Check sheet for the drawn part. Datum: minimum x, y, z corner. Units: mm. A direction names the side the tool comes from. Give positions to 0.01 mm unless a question says otherwise; leave off trailing zeros. Order: outer loops, then holes, each group sorted by start corner. A loop starts at its lowest first (then second) coordinate and runs counter-clockwise, first axis right, second up. Notation, with made-up numbers: M 63.5,14 L 92.5,14 A23 ccw 92.5,45 Z; hole C 56.25,35 d6. An arc over 180 degrees is marked long. One line per question, with ' | ' between items. Start each with the question number.
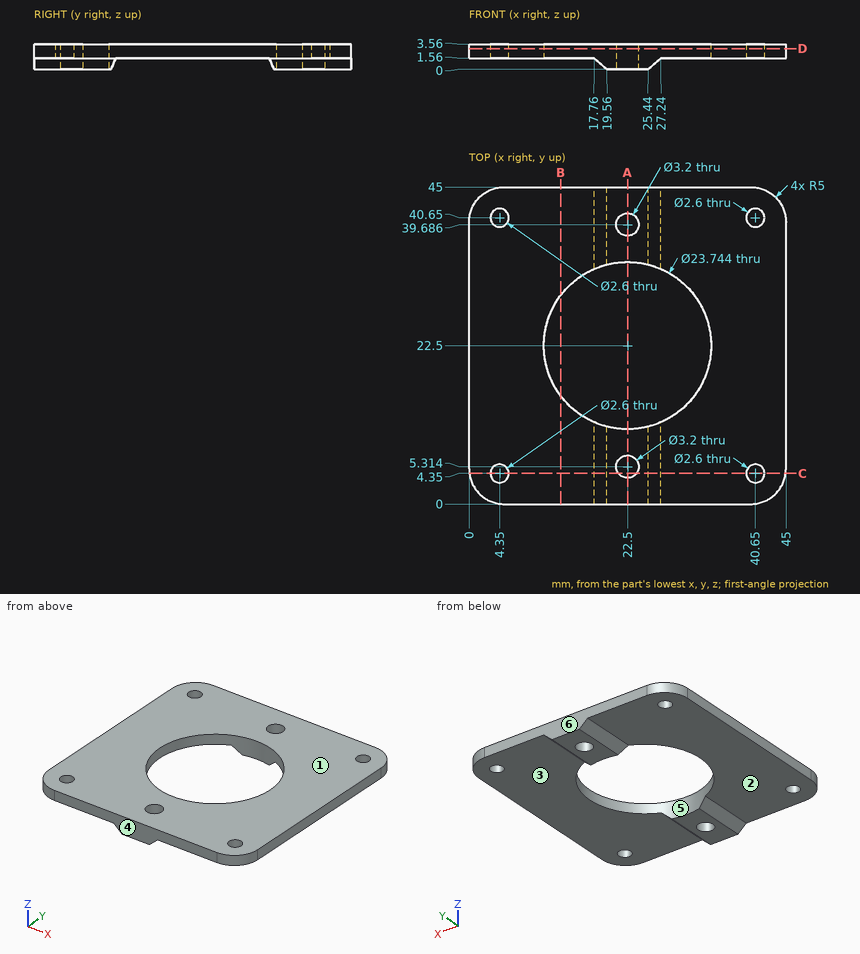
Item 1: Section check D-D, the plane z = 2.9. Record the cut outline in (x, y).
Item 2: Section check C-C, the plane y = 4.35. Record the cut outline in (x, z).
Item 3: Set-up check for the marked faces 1 and 2: record each of +Z, -Z, +X, -X, +Y, -Y from which the full face is reachable in a straight line by a thin tool's end or side.
Item 4: Scan lines: probe 1 along Y at (x, z) = (22.5, 1.4); probe 2 along Y at (x, z) = (4.35, 3.05); probe 3 along X at (y, z) = (22.5, 2.5). Record each from-to range of solid material in increasing order. Write a range as [from, to].
Item 5: Draft check along Y on the marked faces 3, 4, 5 and 6. Enter one of: released by +Y, released by -Y, zero draft, split by the parting line, or undercut.
Item 6: Go/stop test with flat-tipped pins: P1, Ø4, axis at x = 4.35, y = 40.65, coming from the -Z side; P2, Ø1.9, axis at x = 22.5, y = 5.314, coming from the +Z side. Record where each tip stops, or that it passes through.
Item 7: Section check A-A, the plane x = 22.5. Record the cut outline in (y, z), then the cut area to 3 significant figures.
Item 8: Section check B-B, the plane x = 13. Record the cut outline in (y, z).
Reported:
1) outline: M 0,5 A5 ccw 5,0 L 40,0 A5 ccw 45,5 L 45,40 A5 ccw 40,45 L 5,45 A5 ccw 0,40 Z; hole C 4.35,4.35 d2.6; hole C 4.35,40.65 d2.6; hole C 22.5,22.5 d23.74; hole C 22.5,5.31 d3.2; hole C 22.5,39.69 d3.2; hole C 40.65,4.35 d2.6; hole C 40.65,40.65 d2.6
2) outline: M 0.04,1.56 L 3.05,1.56 L 3.05,3.56 L 0.04,3.56 Z; M 5.65,1.56 L 17.76,1.56 L 19.56,0 L 21.22,0 L 21.22,3.56 L 5.65,3.56 Z; M 23.78,0 L 25.44,0 L 27.24,1.56 L 39.35,1.56 L 39.35,3.56 L 23.78,3.56 Z; M 41.95,1.56 L 44.96,1.56 L 44.96,3.56 L 41.95,3.56 Z
3) face 1: +Z, +X, -X, +Y, -Y | face 2: -Z, -X, +Y, -Y
4) probe 1: y = [0, 3.71], [6.91, 10.63], [34.37, 38.09], [41.29, 45] | probe 2: y = [0.04, 3.05], [5.65, 39.35], [41.95, 44.96] | probe 3: x = [0, 10.63], [34.37, 45]
5) face 3: zero draft | face 4: released by -Y | face 5: undercut | face 6: released by +Y
6) P1: stops at z = 1.56 | P2: passes through
7) outline: M 0,0 L 3.71,0 L 3.71,3.56 L 0,3.56 Z; M 6.91,0 L 10.63,0 L 10.63,3.56 L 6.91,3.56 Z; M 34.37,0 L 38.09,0 L 38.09,3.56 L 34.37,3.56 Z; M 41.29,0 L 45,0 L 45,3.56 L 41.29,3.56 Z | area: 52.9 mm^2
8) outline: M 0,1.56 L 15.38,1.56 L 15.38,3.56 L 0,3.56 Z; M 29.62,1.56 L 45,1.56 L 45,3.56 L 29.62,3.56 Z
